Part model, mm, in its own coordinate system. A direction names the side the tool comes from. Coordinates: 2 decimals unless noted, no trailing zeros. Order: outer loops, then holes, each group sorted by start corner. A loop starts at its lowest first (then second) coordinate and runs counter-clockwise, first axis right, second up.
from build123d import *

# Parameters (mm, degrees)
F0_R     = 10
F0_W     = 4.646443
F0_H     = 1.266593
F0_R_2   = 1.5
F1_DEPTH = 6


with BuildPart() as f1:
    # F0 (on Top) → F1 (new body)
    with BuildSketch(Plane.XY):
        Circle(F0_R)
        with Locations((-4.260709, -5.35391)):
            Rectangle(F0_W, F0_H, mode=Mode.SUBTRACT)
        Circle(F0_R_2, mode=Mode.SUBTRACT)
    extrude(amount=F1_DEPTH)


solid = f1.part
Q1. Which spindle directions (+Z, -Z, +X, -X, +Y, -Y) get a long thin tool onto all of the face, cutting with end or side? Do faces 1 (the face through (-1.937, -5, 3)), 2 (the face through (2, 0, 6)). Say none if no direction does.
Results list:
face 1: +Z, -Z
face 2: +Z, +X, -X, +Y, -Y
Q2. Cut at A-A on y = 0. Write the cut outline in (x, z), and give its area (3 significant figures).
Results list:
outline: (-10, 0) - (-1.5, 0) - (-1.5, 6) - (-10, 6) - close; (1.5, 0) - (10, 0) - (10, 6) - (1.5, 6) - close
area: 102 mm2
Q3. Mould opens along Y. For faces 3 (the face through (2, 0, 0)), 4 (the face through (-2.17, -9.76, 2.96)), 5 (the face through (-4, -4.721, 3)) say: pulls with the +Y half, pulls with the -Y half, needs draft (parallel to the pull), parting line crosses it, or undercut.
Results list:
face 3: needs draft
face 4: parting line crosses it
face 5: undercut
Q4. Cut at C-C on z = 1.55. Write the cut outline in (x, y), and give its area (3 significant figures).
Results list:
outline: circle Ø20 at (0, 0); hole (-6.58, -5.99) - (-1.94, -5.99) - (-1.94, -4.72) - (-6.58, -4.72) - close; hole circle Ø3 at (0, 0)
area: 301 mm2
Q5. Wall check: line 1 along Y through (x, z) = (0, 3.9); line 2 along Y through (x, z) = (-3.5, 1.55); line 3 along X through (y, z) = (-0.5, 1.95). Give the ranges that are in metal, low to high.
Results list:
line 1: y = -10 to -1.5, 1.5 to 10
line 2: y = -9.37 to -5.99, -4.72 to 9.37
line 3: x = -9.99 to -1.41, 1.41 to 9.99
Q6. Cut at D-D on y = -6.75. Write the cut outline in (x, z), and give its area (3 significant figures).
Results list:
outline: (-7.38, 0) - (7.38, 0) - (7.38, 6) - (-7.38, 6) - close
area: 88.5 mm2
Q7. Pin check, flat tips, straight feed: pin 1 Ø3.5 at (x, y) = (0, 0) entering from +Z; pin 2 Ø2.5 at (x, z) = (-3, 2) entering from +Y; pin 3 Ø2.5 at (x, z) = (-4, 2.5) entering from -Y; pin 4 Ø1.5 at (y, z) = (-4.5, 0.5) entering from +X. Stop position of each tip, or through.
Results list:
pin 1: stops at z = 6
pin 2: stops at y = 9.85
pin 3: stops at y = -9.61
pin 4: stops at x = 9.27
